from build123d import *

# Parameters (mm, degrees)
SKETCH_1_W          = 20
SKETCH_1_H          = 20
SKETCH_1_W_2        = 16
SKETCH_1_H_2        = 16
EXTRUDE_1_DEPTH     = 580
SKETCH_2_R          = 2.1
CUT_EXTRUDE_1_DEPTH = 20
SKETCH_3_R          = 2.1
CUT_EXTRUDE_2_DEPTH = 581.689245638


with BuildPart() as part:
    # 草图1 → 凸台-拉伸1 (new body)
    with BuildSketch(Plane.XY):
        Rectangle(SKETCH_1_W, SKETCH_1_H)
        Rectangle(SKETCH_1_W_2, SKETCH_1_H_2, mode=Mode.SUBTRACT)
    extrude(amount=EXTRUDE_1_DEPTH)

    # 草图2 → 切除-拉伸1 (cut)
    with BuildSketch(Plane(origin=(0, 10, 0), x_dir=(1, 0, 0), z_dir=(0, 1, 0))):
        with Locations(Location((0, -10, 0), (0, 0, 270))):
            Circle(SKETCH_2_R)
        with Locations(Location((0, -190, 0), (0, 0, 270))):
            Circle(SKETCH_2_R)
    cut_extrude_1 = extrude(amount=-CUT_EXTRUDE_1_DEPTH, mode=Mode.SUBTRACT)

    # 镜向1: 切除-拉伸1 across plane
    add(cut_extrude_1.mirror(Plane.XY.offset(290)), mode=Mode.SUBTRACT)

    # 草图3 → 切除-拉伸2 (cut, through all)
    with BuildSketch(Plane(origin=(10, 10, 580), x_dir=(0, 0, -1), z_dir=(1, 0, 0))):
        with Locations((10, -10)):
            Circle(SKETCH_3_R)
        with Locations((570, -10)):
            Circle(SKETCH_3_R)
        with Locations((190, -10)):
            Circle(SKETCH_3_R)
        with Locations(Location((390, -10, 0), (0, 0, 180))):
            Circle(SKETCH_3_R)
    extrude(amount=-CUT_EXTRUDE_2_DEPTH, mode=Mode.SUBTRACT)


solid = part.part
Here's how the part is built. I have some questions about the finished solid (model axes, mm). A direction names the side the tool comes from. Round coordinates to 2 decimals unless told otherwise and drop trailing zeros. Loops run counter-clockwise (first coordinate to the right, second up) from the corner with the lowest first, then second, coordinate; pieces in that order, holes last. Notation, with made-up numbers: (85, 46.5) - (105, 46.5) arc R28 cw to (105, 80.5) - close; hole circle Ø4 at (77.25, 56). An arc over 180 degrees is marked (long way). One line per question, with ' | ' between items. Start each with the question number.
Q1. For faces 5 (the flat face through (0, 10, 286)), 6 (the flat face through (0, 8, 286)), which set-ups out of +Z, -Z, +X, -X, +Y, -Y let a thin tool reach every point of the face, with its end or its side?
Q2. Will these pins go through, and if not, where does the flat tip stop? pin 1 (5 mm diameter, centred on x = 0, z = 390, fed in from -Y); pin 2 (2.5 mm diameter, centred on x = 0, z = 190, fed in from +Y).
Q3. We'd pull the mould along X, two halves only. Please class faces 1 (the flat face through (-9, 0, 0)), 2 (the flat face through (10, 0, 286)), 3 (the flat face through (0, -8, 286)), 4 (the flat face through (8, 0, 286)): +X half, -X half, draft (parallel to the pull), parting line (faces both ways), or undercut.
Q4. I want a section at A-A (z = 337). Write out the boundary of the cut face in (x, y).
Q5. Please list where these lines run through material, in increasing order: line 1 (X direction, y = -5.25, z = 159); line 2 (X direction, y = 9.45, z = 390). Write a range as [from, to].
Response values:
1) face 5: +Z, -Z, +X, -X, +Y | face 6: +Z, -Z
2) pin 1: stops at y = -10 | pin 2: passes through
3) face 1: draft | face 2: +X half | face 3: undercut | face 4: undercut
4) outline: (-10, -10) - (10, -10) - (10, 10) - (-10, 10) - close; hole (-8, -8) - (8, -8) - (8, 8) - (-8, 8) - close
5) line 1: x = [-10, -8], [8, 10] | line 2: x = [-10, -2.1], [2.1, 10]
